The model under review builds one solid part; all positions refer to its coordinate system, in mm. A direction names the side the tool comes from. Give positions to 0.01 mm unless a question says otherwise; leave off trailing zeros. Loops run counter-clockwise (first coordinate to the right, second up) from the corner with the lowest first, then second, coordinate; pieces in that order, holes last. Notation, with made-up numbers: (43, 35) - (72, 35) arc R32 ccw to (72, 69) - close; hole circle Ø10 at (-11.5, 80.25). An arc over 180 degrees is marked (long way). Answer as a JSON object with one key per item and string values.
from build123d import *

# Parameters (mm, degrees)
F0_W     = 76.2
F0_H     = 76.2
F1_DEPTH = 76.2
F3_DEPTH = 12.7


with BuildPart() as f1:
    # F0 (on Front) → F1 (new body)
    with BuildSketch(Plane.XZ):
        with Locations((-1.006738, -6.150359)):
            Rectangle(F0_W, F0_H)
    extrude(amount=F1_DEPTH)

    # F2 (on face) → F3 (join)
    with BuildSketch(Plane.XZ.offset(76.2)):
        Polygon((-12.611179, 24.049623), (-27.142872, -24.627578), (-19.382371, -24.627578), (-16.510986, -5.769558), (-4.637417, -3.984643), (2.502245, -22.377034), (11.523983, -20.650868), align=None)
        Polygon((-6.111912, 0.904474), (-16.27817, -1.035652), (-12.863549, 14.718168), align=None, mode=Mode.SUBTRACT)
    extrude(amount=F3_DEPTH)


solid = f1.part
Q1. For faces 1 (the face through (-23, -82, -24.628)), 2 (the face through (6.95, -82.461, -21.526)), 3 (the face through (-9.535, -82.461, 7.908)), 4 (the face through (-17.967, -82.461, -15.331)), list the 3-axis set-ups (+Z, -Z, +X, -X, +Y, -Y) from which the entire face can be reached by the end or side of a thin tool; tool diameter is ignored.
Results:
{"face 1": "-Z, +X, -X, -Y", "face 2": "-Z, +X, -Y", "face 3": "-Y", "face 4": "-Z, -Y"}
Q2. Consider section B-B, the plane z = 5.5. State the section outline as (x, y) points, plus the area to 3 significant figures.
Results:
{"outline": "(-39.11, -76.2) - (-18.15, -76.2) - (-18.15, -88.9) - (-14.86, -88.9) - (-14.86, -76.2) - (-8.36, -76.2) - (-8.36, -88.9) - (-2.6, -88.9) - (-2.6, -76.2) - (37.09, -76.2) - (37.09, 0) - (-39.11, 0) - close", "area": "5,920 mm^2"}
Q3. To check wall thickness, follow probe 1 along Y at (x, z) = (-13.5, 23); probe 2 along Z at (x, y) = (-7, -83) (3 decimals); probe 3 along X at (y, z) = (-83, 18.5). State the ranges of each line that lie inside material, in increasing order. Write a range as [from, to].
Results:
{"probe 1": "y = [-76.2, 0]", "probe 2": "z = [-4.34, 0.735], [2.721, 13.657]", "probe 3": "x = [-14.27, -9.61]"}
Q4. Consider section D-D, the plane x = -24. State the section outline as (y, z) points.
Results:
{"outline": "(-88.9, -24.63) - (-76.2, -24.63) - (-76.2, -44.25) - (0, -44.25) - (0, 31.95) - (-76.2, 31.95) - (-76.2, -14.1) - (-88.9, -14.1) - close"}
Q5. Consider section A-A, the plane x = -10.5. State the section outline as (y, z) points, plus the area to 3 significant figures.
Results:
{"outline": "(-88.9, -4.87) - (-76.2, -4.87) - (-76.2, -44.25) - (0, -44.25) - (0, 31.95) - (-76.2, 31.95) - (-76.2, 20.14) - (-88.9, 20.14) - (-88.9, 9.88) - (-76.2, 9.88) - (-76.2, 0.07) - (-88.9, 0.07) - close", "area": "6,000 mm^2"}
Q6. Consider section C-C, the plane x = 1. State the section outline as (y, z) points, plus the area to 3 significant figures.
Results:
{"outline": "(-88.9, -18.51) - (-76.2, -18.51) - (-76.2, -44.25) - (0, -44.25) - (0, 31.95) - (-76.2, 31.95) - (-76.2, -1.16) - (-88.9, -1.16) - close", "area": "6,030 mm^2"}
Q7. The part is to be moulded in two halves that separate along Z. For faces 5 (the face through (-1.1, -82.5, -13.1)), 6 (the face through (-11.12, -82.46, -0.05)), 7 (the face through (-19.775, -82.461, 0.052)), say which applies: +Z half, -Z half, draft (parallel to the pull), parting line (faces both ways), or undercut.
Results:
{"face 5": "-Z half", "face 6": "undercut", "face 7": "+Z half"}
Q8. Clearance check with flat-ended pins moving along their axes: pin 1 Ø3 at (x, z) = (21.5, -22.5) entering from +Y; pin 2 Ø8.5 at (x, y) = (-25, -83.5) entering from -Z. State where each tip first meets the part, or that it passes through.
Results:
{"pin 1": "stops at y = 0", "pin 2": "stops at z = -24.63"}
